The listing builds one solid part. Answer for the finished solid, in the listing's coordinates (mm). Face numbers are marked on the shaded views. A direction names the side the tool comes from. Give positions to 0.01 mm unless a question says otherwise; leave off trailing zeros. Loops run counter-clockwise (first coordinate to the right, second up) from the corner with the lowest first, then second, coordinate; pieces in that order, holes last. Notation, with made-up numbers: (82, 20.5) - (88, 20.5) arc R24 ccw to (88, 46.5) - close; hole circle Ø8 at (43.25, 72). An arc over 180 degrees is marked (long way). One line per item, written item: value. Start each with the question number.
from build123d import *

# Parameters (mm, degrees)
EXTRUDE_1_DEPTH          = 10
FILLET_1_R               = 0.5
SKETCH_2_R               = 2
EXTRUDE_2_DEPTH          = 12.5
EXTRUDE_START            = 0.5
EXTRUDE_3_DEPTH          = 0.5
CUT_EXTRUDE_START        = -0.5
CUT_EXTRUDE_1_DEPTH      = 0.5
FILLET_2_R               = 0.5
HOLE_WIZARD_M31_D        = 2.5
HOLE_WIZARD_M31_DEPTH    = 8.5
HOLE_WIZARD_M31_TIP      = 0.751075774
CUT_EXTRUDE_2_DEPTH      = 10
CUT_EXTRUDE_2_DEPTH_BACK = 10
SKETCH_8_R               = 0.875


with BuildPart() as part:
    # Sketch 1 → Extrude 1 (new body)
    with BuildSketch(Plane.XY):
        with BuildLine():
            Line((2.2, -1.850844402), (2.2, 1.850844402))
            ThreePointArc((2.2, 1.850844402), (-2.875, 0), (2.2, -1.850844402))
        make_face()
    extrude(amount=EXTRUDE_1_DEPTH)

    # Fillet 1
    fillet_1_edges = [part.edges().sort_by_distance(p)[0] for p in [
        (-2.875, 0, 10),
        (2.2, 0, 10),
    ]]
    fillet(fillet_1_edges, radius=FILLET_1_R)

    # Sketch 2 → Extrude 2 (add)
    with BuildSketch(Plane(origin=(0, 0, 0), x_dir=(-1, 0, 0), z_dir=(0, 0, -1))):
        Circle(SKETCH_2_R)
    extrude(amount=EXTRUDE_2_DEPTH)

    # Sketch 3 → Extrude 3 (add)
    with BuildSketch(Plane.XY.offset(-7.25).offset(EXTRUDE_START)):
        with BuildLine():
            Line((2.449489743, -2.5), (1.399708424, -1.428571429))
            ThreePointArc((1.399708424, -1.428571429), (-2, 0), (1.399708424, 1.428571429))
            Line((1.399708424, 1.428571429), (2.449489743, 2.5))
            ThreePointArc((2.449489743, 2.5), (-3.5, 0), (2.449489743, -2.5))
        make_face()
    extrude(amount=-EXTRUDE_3_DEPTH)

    # Sketch 4 → Cut-Extrude 1 (cut)
    with BuildSketch(Plane(origin=(0, 0, -7.25), x_dir=(-1, 0, 0), z_dir=(0, 0, -1)).offset(CUT_EXTRUDE_START)):
        with BuildLine():
            Line((1.944543648, -1.767766953), (1.767766953, -1.944543648))
            ThreePointArc((1.767766953, -1.944543648), (1.237436867, -2.164213562), (0.707106781, -1.944543648))
            Line((0.707106781, -1.944543648), (0.652968438, -1.890405305))
            ThreePointArc((0.652968438, -1.890405305), (1.414213562, -1.414213562), (1.890405305, -0.652968438))
            Line((1.890405305, -0.652968438), (1.944543648, -0.707106781))
            ThreePointArc((1.944543648, -0.707106781), (2.164213562, -1.237436867), (1.944543648, -1.767766953))
        make_face()
        with BuildLine():
            Line((1.767766953, 1.944543648), (1.944543648, 1.767766953))
            ThreePointArc((1.944543648, 1.767766953), (2.164213562, 1.237436867), (1.944543648, 0.707106781))
            Line((1.944543648, 0.707106781), (1.890405305, 0.652968438))
            ThreePointArc((1.890405305, 0.652968438), (1.414213562, 1.414213562), (0.652968438, 1.890405305))
            Line((0.652968438, 1.890405305), (0.707106781, 1.944543648))
            ThreePointArc((0.707106781, 1.944543648), (1.237436867, 2.164213562), (1.767766953, 1.944543648))
        make_face()
    extrude(amount=CUT_EXTRUDE_1_DEPTH, mode=Mode.SUBTRACT)

    # Fillet 2
    fillet_2_edges = [part.edges().sort_by_distance(p)[0] for p in [
        (2.449489743, 2.5, -7),
        (2.449489743, -2.5, -7),
    ]]
    fillet(fillet_2_edges, radius=FILLET_2_R)

    # Hole Wizard M31
    with Locations(Plane(origin=(0, 0, -12.5), x_dir=(-1, 0, 0), z_dir=(0, 0, -1))):
        with Locations((0, 0)):
            Hole(HOLE_WIZARD_M31_D / 2, depth=HOLE_WIZARD_M31_DEPTH)
            with Locations((0, 0, -(HOLE_WIZARD_M31_DEPTH + HOLE_WIZARD_M31_TIP / 2))):  # 118° drill point
                Cone(0, HOLE_WIZARD_M31_D / 2, HOLE_WIZARD_M31_TIP, mode=Mode.SUBTRACT)

    # Sketch 8 → Cut-Extrude 2 (cut, two sides: drawn at the far end of the back side and taken through both)
    with BuildSketch(Plane(origin=(0, 0, 0), x_dir=(1, 0, 0), z_dir=(0, 1, 0)).offset(-CUT_EXTRUDE_2_DEPTH_BACK)):
        with Locations(Location((0, 10, 0), (0, 0, 90))):
            Circle(SKETCH_8_R)
    extrude(amount=CUT_EXTRUDE_2_DEPTH + CUT_EXTRUDE_2_DEPTH_BACK, mode=Mode.SUBTRACT)


solid = part.part
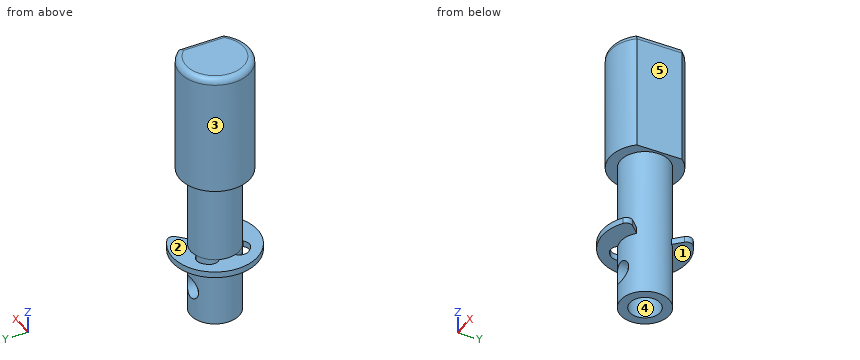
1. Find the intervals of material crossed by L1, parallel to Y at x = 0, z = -5.75; L2, parallel to X at y = -1, z = -5.5; L3, parallel to X at y = 0, z = 7 (3 decimals), in increasing order. Write a range as [from, to].
2. Flat-ended cylindrical pins translate along their axes: pin 1 (1.4 mm diameter, centred on x = 0, z = -10, fed in from -Y); pin 2 (2 mm diameter, centred on x = -1.5, z = -8.5, fed in from +Y); pin 3 (3 mm diameter, centred on y = 0.5, z = 6.5, fed in from +X); pin 4 (2.5 mm diameter, centred on x = 0, z = -10, fed in from +Y). Find the tip coordinate at first contact, or state that the pin passes through.
3. A cutting plane is placed at B-B (x = -1.45). Give the number of separate pieces and of enclosed holes in the cut face, plus the area to 3 significant figures.
4. Determine the mould class of the marked faces 1, 2 and 3 for opening direction Z: released by +Z, released by -Z, zero draft, split by the parting line, or undercut.
5. A cutting plane is placed at A-A (z = -10). Determine the outline of the cut face in (x, y) (3 decimals), plus the area to 3 significant figures.
6. For the marked faces 4 and 5, determine the directions among +Z, -Z, +X, -X, +Y, -Y from which every point of the face is accessible in a straight line to the end or side of a thin tool.
7. A cutting plane is placed at C-C (z = 0.5). Determine the outline of the cut face in (x, y) (3 decimals).
Results below:
1. L1: y = [-2, -1.25], [1.25, 2]
1. L2: x = [-1.73, -0.75], [0.75, 1.73]
1. L3: x = [-2.875, 2.2]
2. pin 1: passes through
2. pin 2: stops at y = 1.94
2. pin 3: stops at x = 2.2
2. pin 4: stops at y = 2
3. separate pieces: 3
3. enclosed holes: 0
3. area: 85.0 mm^2
4. face 1: released by -Z
4. face 2: undercut
4. face 3: zero draft
5. outline: (-0.875, -1.798) - (-0.875, -0.893) arc R1.25 cw to (-0.875, 0.893) - (-0.875, 1.798) arc R2 ccw to start; (0.875, -1.798) arc R2 ccw to (0.875, 1.798) - (0.875, 0.893) arc R1.25 cw to (0.875, -0.893) - close
5. area: 4.87 mm^2
6. face 4: -Z
6. face 5: +Z, -Z, +X, +Y, -Y
7. outline: (2.2, -1.851) - (2.2, 1.851) arc R2.875 ccw (long way) to start
